```python
from build123d import *

# Parameters (mm, degrees)
CROQUIS1_W              = 200
CROQUIS1_H              = 300
SALIENTE_EXTRUIR1_DEPTH = 5
CROQUIS2_R              = 11
CORTAR_EXTRUIR1_DEPTH   = 15
CROQUIS3_R              = 2
AG_COLUMNA_DEPTH        = 15
CROQUIS4_R              = 2
CORTAR_EXTRUIR3_DEPTH   = 15
CROQUIS5_R              = 3
CROQUIS5_W              = 20
CROQUIS5_H              = 35
CROQUIS5_W_2            = 35
CROQUIS5_H_2            = 20
CORTAR_EXTRUIR4_DEPTH   = 1.7
CROQUIS6_W              = 30.5
CROQUIS6_H              = 30.5
CORTAR_EXTRUIR5_DEPTH   = 2.5


with BuildPart() as part:
    # Croquis1 → Saliente-Extruir1 (new body)
    with BuildSketch(Plane.XY):
        Rectangle(CROQUIS1_W, CROQUIS1_H)
    extrude(amount=SALIENTE_EXTRUIR1_DEPTH)

    # Croquis2 → Cortar-Extruir1 (cut)
    with BuildSketch(Plane.XY.offset(5)):
        with Locations((0, 120)):
            Circle(CROQUIS2_R)
    extrude(amount=-CORTAR_EXTRUIR1_DEPTH, mode=Mode.SUBTRACT)

    # Croquis3 → Ag. Columna (cut)
    with BuildSketch(Plane.XY.offset(5)):
        with Locations((85, 135)):
            Circle(CROQUIS3_R)
        with Locations((-85, 135)):
            Circle(CROQUIS3_R)
        with Locations((-85, -135)):
            Circle(CROQUIS3_R)
        with Locations((85, -135)):
            Circle(CROQUIS3_R)
    extrude(amount=-AG_COLUMNA_DEPTH, mode=Mode.SUBTRACT)

    # Croquis4 → Cortar-Extruir3 (cut)
    with BuildSketch(Plane.XY.offset(5)):
        with Locations((-50, 6)):
            Circle(CROQUIS4_R)
        with Locations(Location((-50, -6, 0), (0, 0, 180))):
            Circle(CROQUIS4_R)
        with Locations((50, -7)):
            Circle(CROQUIS4_R)
        with Locations(Location((50, 7, 0), (0, 0, 180))):
            Circle(CROQUIS4_R)
        with Locations((-7.668433443, 75)):
            Circle(CROQUIS4_R)
        with Locations(Location((7.668433443, 75, 0), (0, 0, 180))):
            Circle(CROQUIS4_R)
        with Locations(Location((-7.668433443, -75, 0), (0, 0, 180))):
            Circle(CROQUIS4_R)
        with Locations((7.668433443, -75)):
            Circle(CROQUIS4_R)
    extrude(amount=-CORTAR_EXTRUIR3_DEPTH, mode=Mode.SUBTRACT)

    # Croquis5 → Cortar-Extruir4 (cut)
    with BuildSketch(Plane.XY.offset(5)):
        with Locations((-85, 135)):
            Circle(CROQUIS5_R)
        with Locations(Location((85, 135, 0), (0, 0, 180))):
            Circle(CROQUIS5_R)
        with Locations(Location((-85, -135, 0), (0, 0, 180))):
            Circle(CROQUIS5_R)
        with Locations((85, -135)):
            Circle(CROQUIS5_R)
        with Locations((-50, 0)):
            Rectangle(CROQUIS5_W, CROQUIS5_H)
        with Locations((0, -75.070372891)):
            Rectangle(CROQUIS5_W_2, CROQUIS5_H_2)
        with Locations((0, 75.070372891)):
            Rectangle(CROQUIS5_W_2, CROQUIS5_H_2)
        with Locations((50, 0)):
            Rectangle(CROQUIS5_W, CROQUIS5_H)
    extrude(amount=-CORTAR_EXTRUIR4_DEPTH, mode=Mode.SUBTRACT)

    # Croquis6 → Cortar-Extruir5 (cut)
    with BuildSketch(Plane(origin=(0, 0, 0), x_dir=(-1, 0, 0), z_dir=(0, 0, -1))):
        with Locations((-84.75, 134.75)):
            Rectangle(CROQUIS6_W, CROQUIS6_H)
        with Locations((84.75, 134.75)):
            Rectangle(CROQUIS6_W, CROQUIS6_H)
        with Locations((84.75, -134.75)):
            Rectangle(CROQUIS6_W, CROQUIS6_H)
        with Locations((-84.75, -134.75)):
            Rectangle(CROQUIS6_W, CROQUIS6_H)
    extrude(amount=-CORTAR_EXTRUIR5_DEPTH, mode=Mode.SUBTRACT)


solid = part.part
```
Work out the finished part from the listing and answer in its coordinate system (mm). A direction names the side the tool comes from. Give positions to 0.01 mm unless a question says otherwise; leave off trailing zeros. Order: outer loops, then holes, each group sorted by start corner. A loop starts at its lowest first (then second) coordinate and runs counter-clockwise, first axis right, second up. Notation, with made-up numbers: (65, 22) - (110, 22) arc R21 ccw to (110, 47) - close; hole circle Ø2 at (71.5, 2). An arc over 180 degrees is marked (long way). One line per item, written item: value. Start each with the question number.
1. Consider line 1 (X direction, y = 135, z = 2.7); line 2 (Y direction, x = -50, z = 1.4); line 3 (Y direction, x = 50, z = 1.3). Determine where each line is inside the solid, lowest interval first.
2. Which of the six approach directions +Z, -Z, +X, -X, +Y, -Y give full straight-line access (tool end or side, diameter ignored) to faces 3 (the face through (88, 135, 2.5)), 4 (the face through (-81, 135, 2.5)), 5 (the face through (50, 0, 3.3)), 6 (the face through (88, -135, 2.5)), 7 (the face through (-1, 2, 5))?
3. Each of these flat-tipped pins is pushed along its axis until it touches: pin 1 Ø8 at (x, y) = (-85, 135) entering from -Z; pin 2 Ø6 at (x, y) = (-2.5, 70.5) entering from +Z. Where does it stop, or does it pass through?
4. For a pull along Y with two mould halves and no side action, classify faces 1 (the face through (-81, -135, 2.5)), 2 (the face through (0, -75, 3.3)) as released by +Y, released by -Y, zero draft, split by the parting line, or undercut.
5. Section D-D, the plane y = 112 is taken. Write down the section's boundary in (x, z).
6. Section B-B, the plane y = -123.5 is taken. Write down the section's boundary in (x, z).
7. Section A-A, the plane z = 1.55 is taken. Count the separate pieces of the cut face and the enclosed holes in it, then the cut area to 3 significant figures.
8. Section C-C, the plane x = 57 is taken. Write down the section's boundary in (y, z).
Filled sheet:
1. line 1: -100 to -87, -83 to 83, 87 to 100
1. line 2: -150 to -8, -4 to 4, 8 to 150
1. line 3: -150 to -9, -5 to 5, 9 to 150
2. face 3: -Z, +X, +Y
2. face 4: -Z, -X, +Y
2. face 5: +Z
2. face 6: -Z, +X, -Y
2. face 7: +Z, +X, -X, +Y, -Y
3. pin 1: z = 2.5
3. pin 2: z = 3.3
4. face 1: zero draft
4. face 2: undercut
5. outline: (-100, 0) - (-7.55, 0) - (-7.55, 5) - (-100, 5) - close; (7.55, 0) - (100, 0) - (100, 5) - (7.55, 5) - close
6. outline: (-100, 2.5) - (-69.5, 2.5) - (-69.5, 0) - (69.5, 0) - (69.5, 2.5) - (100, 2.5) - (100, 5) - (-100, 5) - close
7. separate pieces: 1
7. enclosed holes: 9
7. area: 55,800 mm²
8. outline: (-150, 0) - (150, 0) - (150, 5) - (17.5, 5) - (17.5, 3.3) - (-17.5, 3.3) - (-17.5, 5) - (-150, 5) - close
